Autodesk Inventor part; units mm, degrees
ref_plane "YZ Plane" through (0, 0, 0) normal (1, 0, 0) x (0, 1, 0)
ref_plane "XZ Plane" through (0, 0, 0) normal (0, 1, 0) x (-1, 0, 0)
ref_plane "XY Plane" through (0, 0, 0) normal (0, 0, 1) x (1, 0, 0)
sketch "Sketch1" plane through (0, 0, 0) normal (0, 1, 0) x (-1, 0, 0)
  line L0 (3.9336, 17.4729) -> (3.9336, -2.5271)
  line L1 (3.9336, -2.5271) -> (13.9336, -2.5271)
  line L2 (13.9336, -2.5271) -> (13.9336, -57.5271)
  line L3 (13.9336, -57.5271) -> (3.9336, -57.5271)
  line L4 (3.9336, -57.5271) -> (3.9336, -77.5271)
  line L5 (3.9336, -77.5271) -> (23.9336, -77.5271)
  line L6 (23.9336, -77.5271) -> (23.9336, -57.5271)
  line L7 (3.9336, 17.4729) -> (63.9336, 17.4729)
  line L8 (63.9336, 17.4729) -> (63.9336, -2.5271)
  line L9 (63.9336, -2.5271) -> (53.9336, -2.5271)
  line L10 (53.9336, -2.5271) -> (53.9336, -22.5271)
  arc A0 (53.9336, -22.5271) -> (23.9336, -57.5271) centre (59.3503, -57.5271) ccw
  point P0 (0, 0)
  dimension "d0" = 20
  dimension "d1" = 10
  dimension "d2" = 55
  dimension "d3" = 10
  dimension "d4" = 20
  dimension "d5" = 20
  dimension "d6" = 20
  dimension "d7" = 60
  dimension "d8" = 20
  dimension "d9" = 10
  dimension "d10" = 20
extrude "Extrusion1" add sketch "Sketch1" along normal blind 5
sketch "Sketch2" plane through (0, 5, 0) normal (0, 1, 0) x (1, 0, 0)
  circle A0 centre (-13.9336, -7.4729) radius 5.25
  circle A1 centre (-13.9336, 67.5271) radius 5.25
  circle A2 centre (-53.9336, -7.4729) radius 3.25
  point P0 (0, 0)
  point P1 (-3.9336, -17.4729)
  point P2 (-3.9336, 77.5271)
  dimension "d15" = 10.5
  dimension "d18" = 10.5
  dimension "d21" = 6.5
extrude "Extrusion2" cut sketch "Sketch2" along normal through all both and the other way through all
sketch "Sketch3" plane through (0, 5, 0) normal (0, 1, 0) x (1, 0, 0)
  line L0 (-63.9336, -17.4729) -> (-3.9336, -17.4729)
  line L1 (-13.9336, 2.5271) -> (-13.9336, 57.5271)
  circle A0 centre (-25.9336, 17.5271) radius 2.5
  point P0 (0, 0)
  dimension "d27" = 5
extrude "Extrusion3" cut sketch "Sketch3" against normal through all
fillet "Fillet1" radius 4 2 edges at (-13.9336, 2.5, -2.5271) (-23.9336, 2.5, -77.5271)
fillet "Fillet2" radius 2 7 edges at (-3.9336, 2.5, 17.4729) (-63.9336, 2.5, 17.4729) (-3.9336, 2.5, -2.5271) (-3.9336, 2.5, -57.5271) (-3.9336, 2.5, -77.5271) (-63.9336, 2.5, -2.5271) (-53.9336, 2.5, -22.5271)
fillet "Fillet3" radius 2 2 edges at (-13.9336, 2.5, -57.5271) (-53.9336, 2.5, -2.5271)
properties part number "autodesk"
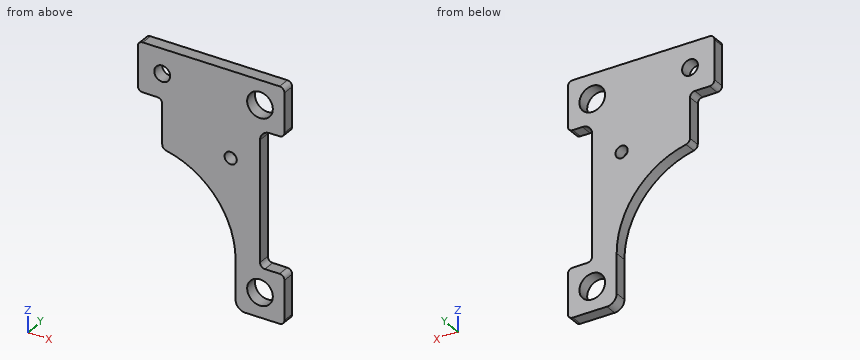
CAD build for the part. Positions are in the model's coordinates, mm. Give positions to 0.01 mm unless a question says otherwise; leave off trailing zeros. Write each loop counter-clockwise with the first axis right and the second up, starting at its lowest first coordinate (ties: lowest second). Pieces come first, ordered by that corner, then holes. Notation, with made-up numbers: M -20,43 L 6,43 A16 ccw 6,53 Z; hole C -17.5,3.25 d8. An arc over 180 degrees is marked long. Return JSON: item names as keys, results as strings. Group by question number.
(1) Band-saw the part on D-D (y = 0.75). Give the cut face in (x, z).
(2) Flat gauge pins, fed straight in: pin 1 Ø8.5 at (x, z) = (-13.93, -67.53) entering from +Y; pin 2 Ø2.5 at (y, z) = (3, -16) entering from -X; pin 3 Ø12 at (x, z) = (-13.93, 7.47) entering from -Y; pin 4 Ø2.5 at (x, y) = (-57.5, 1.5) entering from -Z. Where does each tip first touch, or does it go through?
(3) Drill centre lines: L1, parallel to Z at x = -6, y = 2.35; L2, parallel to Z at x = -11, y = 2.4; L3, parallel to Z at x = -16.5, y = 3.9. Where is each one in solid material? Low to high. Write a range as [from, to].
(4) Band-saw the part on B-B (x = -13). Give the cut face in (y, z).
(5) Band-saw the part on C-C (x = -26). Give the cut face in (y, z), and give its area (3 significant figures).
(6) Band-saw the part on A-A (z = -71.5). Give the cut face in (x, y).
Entries:
{
 "1": {"outline": "M -63.93,-0.53 A2 ccw -61.93,-2.53 L -55.93,-2.53 A2 cw -53.93,-4.53 L -53.93,-20.85 A2 ccw -52.33,-22.81 A35.42 cw -23.93,-57.53 L -23.93,-73.53 A4 ccw -19.93,-77.53 L -5.93,-77.53 A2 ccw -3.93,-75.53 L -3.93,-59.53 A2 ccw -5.93,-57.53 L -11.93,-57.53 A2 cw -13.93,-55.53 L -13.93,-6.53 A4 cw -9.93,-2.53 L -5.93,-2.53 A2 ccw -3.93,-0.53 L -3.93,15.47 A2 ccw -5.93,17.47 L -61.93,17.47 A2 ccw -63.93,15.47 Z; hole C -53.93,7.47 d6.5; hole C -25.93,-17.53 d5; hole C -13.93,-67.53 d10.5; hole C -13.93,7.47 d10.5"},
 "2": {"pin 1": "passes through", "pin 2": "stops at x = -53.93", "pin 3": "stops at y = 0", "pin 4": "stops at z = -2.53"},
 "3": {"L1": "z = [-77.53, -57.53], [-2.53, 17.47]", "L2": "z = [-77.53, -71.88], [-63.17, -57.53], [-2.67, 3.12], [11.83, 17.47]", "L3": "z = [-77.53, -72.11], [-62.95, 2.89], [12.05, 17.47]"},
 "4": {"outline": "M 0,-77.53 L 5,-77.53 L 5,-72.69 L 0,-72.69 Z; M 0,-62.36 L 5,-62.36 L 5,-57.22 L 0,-57.22 Z; M 0,-3.96 L 5,-3.96 L 5,2.31 L 0,2.31 Z; M 0,12.64 L 5,12.64 L 5,17.47 L 0,17.47 Z"},
 "5": {"outline": "M 0,-45.61 L 5,-45.61 L 5,-20.03 L 0,-20.03 Z; M 0,-15.03 L 5,-15.03 L 5,17.47 L 0,17.47 Z", "area": "290 mm^2"},
 "6": {"outline": "M -23.93,0 L -17.37,0 L -17.37,5 L -23.93,5 Z; M -10.5,0 L -3.93,0 L -3.93,5 L -10.5,5 Z"}
}
